Input: part model. Units: mm. Frame: model coordinates. A direction names the side the tool comes from. Round coordinates to 2 decimals unless told otherwise and drop trailing zeros. Write each loop counter-clockwise with the first axis right and the second up, starting at its lowest first coordinate (ties: lowest second). Pieces come first, ordered by that corner, then holes. Notation, with made-up numbers: (87.25, 43.5) - (92.25, 43.5) arc R15 cw to (92.25, 60.5) - close; hole circle Ø11 at (54, 20.5). An arc over 180 degrees is marked (long way). Use one line per item in the form item = value.
```python
from build123d import *

# Parameters (mm, degrees)
F0_W     = 152.4
F0_H     = 152.4
F1_DEPTH = 127
F0_H_2   = 25.4
F0_W_2   = 25.4
F2_DEPTH = 50.8
F3_T     = -12.7


with BuildPart() as f1:
    # F0 (on Front) → F1 (new body)
    with BuildSketch(Plane.XZ):
        with Locations((12.7657866001, 13.8525208354)):
            Rectangle(F0_W, F0_H)
    extrude(amount=F1_DEPTH)

    # F0 (on Front) → F2 (join)
    with BuildSketch(Plane.XZ):
        with Locations((12.7657866001, 102.7525208354)):
            Rectangle(F0_W, F0_H_2)
        with Locations((-76.1342133999, 13.8525208354)):
            Rectangle(F0_W_2, F0_H)
        with Locations((-76.1342133999, 102.7525208354)):
            Rectangle(F0_W_2, F0_H_2)
        with Locations((12.7657866001, -75.0474791646)):
            Rectangle(F0_W, F0_H_2)
        with Locations((-76.1342133999, -75.0474791646)):
            Rectangle(F0_W_2, F0_H_2)
        with Locations((101.6657866001, 13.8525208354)):
            Rectangle(F0_W_2, F0_H)
        with Locations((101.6657866001, 102.7525208354)):
            Rectangle(F0_W_2, F0_H_2)
        with Locations((101.6657866001, -75.0474791646)):
            Rectangle(F0_W_2, F0_H_2)
    extrude(amount=F2_DEPTH)

    # F3
    f3_openings = [f1.faces().sort_by_distance(p)[0] for p in [
        (12.765787, -127, 13.852521),
    ]]
    offset(amount=F3_T, openings=f3_openings, kind=Kind.INTERSECTION)


solid = f1.part
```
(1) Material intervals for L1, parallel to X at y = -109.5, z = 69.5; L2, parallel to Z at x = 71.5, y = -21; L3, parallel to Y at x = 56, z = -69.5, sorted ascending.
Derived:
L1 = -63.43 to -50.73, 76.27 to 88.97
L2 = -87.75 to -75.05, 102.75 to 115.45
L3 = -50.8 to -38.1, -12.7 to 0
(2) Access query for faces 4 (the face through (88.966, -88, 13)), 5 (the face through (-68, -38.1, 15)), 6 (the face through (12, -88, -62.347)). Directions: +Z, -Z, +X, -X, +Y, -Y. A direction counts if a zero-diameter tool reaches every point of the face in a straight line with its end or side. Return the directions, or none.
Derived:
face_4 = +Z, -Z, +X, -Y
face_5 = none
face_6 = -Z, +X, -X, -Y
(3) Cut plane D-D on z = 87.5. Output: boundary loops of the cut face in (x, y), then the cut area to 3 significant figures.
Derived:
outline = (-88.83, -50.8) - (-63.43, -50.8) - (-63.43, -127) - (88.97, -127) - (88.97, -50.8) - (114.37, -50.8) - (114.37, 0) - (-88.83, 0) - close; hole (-76.13, -38.1) - (101.67, -38.1) - (101.67, -12.7) - (-76.13, -12.7) - close
area = 17,400 mm^2
(4) Draft query along Z for faces 1 (the face through (14, -25, 102.753)), 2 (the face through (-79, -50.8, 15)), 3 (the face through (12, -88, 90.053)). Return one class per face: released by +Z, released by -Z, zero draft, split by the parting line, or undercut.
Derived:
face_1 = undercut
face_2 = zero draft
face_3 = released by +Z
(5) Cut plane A-A on x = 92.5. Output: boundary loops of the cut face in (y, z), then the cut area to 3 significant figures.
Derived:
outline = (-50.8, -87.75) - (0, -87.75) - (0, 115.45) - (-50.8, 115.45) - close; hole (-38.1, -75.05) - (-12.7, -75.05) - (-12.7, 102.75) - (-38.1, 102.75) - close
area = 5,810 mm^2
(6) Cut plane B-B on y = -96. Output: boundary loops of the cut face in (x, z).
Derived:
outline = (-63.43, -62.35) - (88.97, -62.35) - (88.97, 90.05) - (-63.43, 90.05) - close; hole (-50.73, -49.65) - (76.27, -49.65) - (76.27, 77.35) - (-50.73, 77.35) - close
(7) First-contact query: pin 1 Ø3 at (x, z) = (5.5, 4) entering from -Y; pin 2 Ø8 at (y, z) = (-86.5, -20.5) entering from +X; pin 3 Ø23 at (x, y) = (-21, -96.5) entering from +Z. Flat tips, straight axial feed; report the tip coordinate or a pass-through.
Derived:
pin_1 = -12.7
pin_2 = 88.97
pin_3 = 90.05
(8) Cut plane C-C on z = -4. Output: boundary loops of the cut face in (x, y).
Derived:
outline = (-88.83, -50.8) - (-63.43, -50.8) - (-63.43, -127) - (-50.73, -127) - (-50.73, -38.1) - (-76.13, -38.1) - (-76.13, -12.7) - (101.67, -12.7) - (101.67, -38.1) - (76.27, -38.1) - (76.27, -127) - (88.97, -127) - (88.97, -50.8) - (114.37, -50.8) - (114.37, 0) - (-88.83, 0) - close
